```python
from build123d import *

# Parameters (mm, degrees)
SKETCH095_W      = 6
SKETCH095_H      = 6
EXTRUDE033_DEPTH = 19.3
SKETCH096_R      = 1.6
HOLE019_DEPTH    = 2.5
HOLE019_TIPS_R   = 1.6


with BuildPart() as part:
    # Sketch095 (on Face6 of BaseFeature009) → Extrude033 (new body)
    with BuildSketch(Plane.XY.offset(2)):
        with Locations((5, -104.299998)):
            Rectangle(SKETCH095_W, SKETCH095_H)
    extrude(amount=EXTRUDE033_DEPTH)

    # Sketch096 (on Face6 of Extrude033) → Hole019 (cut)
    with BuildSketch(Plane.XY.offset(21.3)):
        with Locations((5, -104.300002)):
            Circle(SKETCH096_R)
    extrude(amount=-HOLE019_DEPTH, mode=Mode.SUBTRACT)

    # Hole019 tips → Hole019 tip 1 section 0
    with BuildSketch(Plane.XY.offset(18.8), mode=Mode.PRIVATE) as hole019_tip_1_s0:
        with Locations((5, -104.300002)):
            Circle(HOLE019_TIPS_R)
    loft([hole019_tip_1_s0.sketch, Vertex(5, -104.300002, 17.838623)], mode=Mode.SUBTRACT)


solid = part.part
```
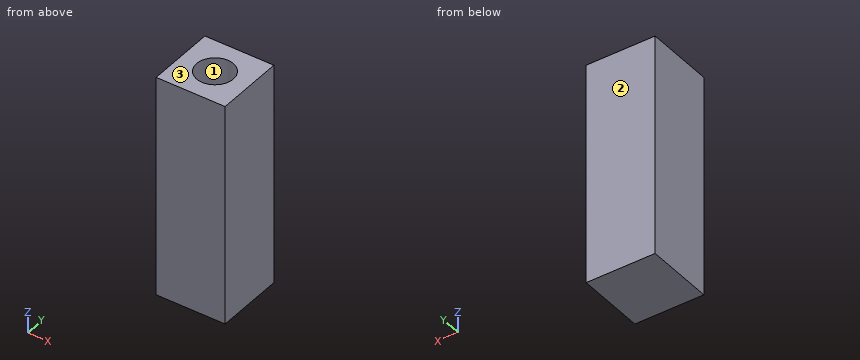
Input: part model. Units: mm. Frame: model coordinates. Face numbers are marked on the shaded views. Round coordinates to 2 decimals unless told otherwise and drop trailing zeros. Write each loop counter-clockwise with the first axis right and the second up, starting at its lowest first coordinate (ties: lowest second). Pieces come first, ordered by that corner, then holes. Notation, with made-up numbers: (-23.5, 65) -> (32.5, 65) arc R26 ccw to (32.5, 84) -> close; hole circle Ø5 at (23.25, 35). An arc over 180 degrees is marked (long way). Answer as CSV lines item,"result".
1. Mould query, pull axis Y, two halves, no side actions, for the marked faces 1, 2 and 3. Classes: +Y half, -Y half, draft (parallel to the pull), parting line (faces both ways), or undercut.
Geometry says:
face 1,"undercut"
face 2,"+Y half"
face 3,"draft"
2. Section A-A (z = 19). Return the cut outline in (x, y).
Geometry says:
outline,"(2, -107.3) -> (8, -107.3) -> (8, -101.3) -> (2, -101.3) -> close; hole circle Ø3.2 at (5, -104.3)"
3. Ray query, L1, parallel to Y at x = 4.9, z = 19.25; L2, parallel to Y at x = 5.85, z = 20; L3, parallel to X at y = -103.05, z = 20.25. Return the intervals inside material, ascending. Write a range as [from, to].
Geometry says:
L1,"y = [-107.3, -105.9], [-102.7, -101.3]"
L2,"y = [-107.3, -105.66], [-102.94, -101.3]"
L3,"x = [2, 4], [6, 8]"
